Could you check a few things on this model? Use its own coordinates, in mm. A direction names the side the tool comes from. Round coordinates to 2 decimals unless told otherwise and drop trailing zeros. Write each loop counter-clockwise with the first axis right and the second up, starting at its lowest first coordinate (ties: lowest second). Pieces come first, ordered by that corner, then holes. Notation, with made-up numbers: (-4.5, 1.25) -> (30.5, 1.25) arc R30 ccw to (30.5, 25.25) -> close; hole circle Ø1 at (80.25, 61.5). An arc over 180 degrees is marked (long way). Answer as CSV lines item,"result". Start each with the question number.
Q1. For faces 4 (the flat face through (79, -133, 177)), 5 (the flat face through (-6.21, -167.31, 172.06)), 6 (the flat face through (77, -151, 0)), which set-ups out of +Z, -Z, +X, -X, +Y, -Y let a thin tool reach every point of the face, with its end or its side?
Q2. Imagine slicing it at C-C on y = -97. Please give me the cut outline in (x, z), and give its area (3 significant figures).
Q3. Imagine slicing it at B-B on z = 26.5. Please give me the cut outline in (x, y).
Q4. Imagine slicing it at A-A on x = 94. Please give me the cut outline in (y, z).
Q5. Will these pins go through, and if not, where does the flat tip stop? pin 1 Ø1 at (x, z) = (186.5, 194) entering from -Y; pin 2 Ø3 at (y, z) = (-92, 281.5) entering from -X; pin 3 Ø2 at (x, z) = (-22.5, 182.5) entering from -Y.
Q6. If we mould it in two halves opening along X, with no side actions, what happens to faces 1 (the flat face through (-47.62, -12.76, 172.06)), 2 (the flat face through (79, 0, 172)), 3 (the flat face through (186.5, -77, 177))? For each: pulls with the +X half, pulls with the -X half, needs draft (parallel to the pull), parting line crosses it, or undercut.
Q7. If I drill on line 1 (X direction, y = -88.5, z = 80); line 2 (X direction, y = -116, z = 50); line 3 (Y direction, x = 145, z = 61), over which ranges is the centre line in solid material (lowest first)? Write a range as [from, to].
Q8. Imagine slicing it at D-D on x = 232.5. Please give me the cut outline in (y, z).
Autodesk Inventor part; units mm, degrees
ref_plane "YZ Plane" through (0, 0, 0) normal (1, 0, 0) x (0, 1, 0)
ref_plane "XZ Plane" through (0, 0, 0) normal (0, 1, 0) x (-1, 0, 0)
ref_plane "XY Plane" through (0, 0, 0) normal (0, 0, 1) x (1, 0, 0)
sketch "Sketch1" plane through (0, 0, 0) normal (0, 0, 1) x (1, 0, 0)
  line L0 (0, 0) -> (160, 0)
  line L1 (160, 0) -> (118.589, -154.5481) construction
  line L2 (0, 0) -> (41.411, -154.5481) construction
  line L3 (41.411, -154.5481) -> (118.589, -154.5481)
  circle A0 centre (235.8871, -103.156) radius 80 construction
  line L4 (160, 0) -> (256.5926, -25.8819)
  line L5 (118.589, -154.5481) -> (215.1815, -180.43)
  arc A1 (215.1815, -180.43) -> (256.5926, -25.8819) centre (235.8871, -103.156) ccw
  circle A2 centre (-75.8871, -103.156) radius 80 construction
  line L6 (0, 0) -> (-96.5926, -25.8819)
  line L7 (41.411, -154.5481) -> (-55.1815, -180.43)
  arc A3 (-96.5926, -25.8819) -> (-55.1815, -180.43) centre (-75.8871, -103.156) ccw
  dimension "d0" = 160
  dimension "d1" = 160
  dimension "d2" = 160
  dimension "d3" = 75
  dimension "d4" = 75
  dimension "d5" = 160
  dimension "d6" = 100
  dimension "d7" = 160
  dimension "d9" = 100
extrude "Extrusion1" add sketch "Sketch1" along normal blind 349
sketch "Sketch2" plane through (0, 0, 349) normal (0, 0, 1) x (1, 0, 0)
  line L0 (-26.5, -133) -> (186.5, -133)
  line L1 (186.5, -133) -> (186.5, -20)
  line L2 (186.5, -20) -> (-26.5, -20)
  line L3 (-26.5, -20) -> (-26.5, -133)
  line L4 (160, 0) -> (0, 0)
  point P0 (80, -20)
  point P1 (80, 0)
  dimension "d12" = 213
  dimension "d13" = 113
  dimension "d14" = 20
extrude "Extrusion2" cut sketch "Sketch2" against normal through all
properties part number "Riser Base" material "ABS Plastic"
Checks:
1,face 4,"+Z, -Z"
1,face 5,"+Z, -Z, -Y"
1,face 6,"-Z, +X, -X, +Y, -Y"
2,outline,"(-155.65, 0) -> (-26.5, 0) -> (-26.5, 349) -> (-155.65, 349) -> close; (186.5, 0) -> (315.65, 0) -> (315.65, 349) -> (186.5, 349) -> close"
2,area,"90,100 mm^2"
3,outline,"(-96.59, -25.88) arc R80 ccw to (-55.18, -180.43) -> (41.41, -154.55) -> (118.59, -154.55) -> (215.18, -180.43) arc R80 ccw to (256.59, -25.88) -> (160, 0) -> (0, 0) -> close; hole (-26.5, -133) -> (186.5, -133) -> (186.5, -20) -> (-26.5, -20) -> close"
4,outline,"(-154.55, 0) -> (-133, 0) -> (-133, 349) -> (-154.55, 349) -> close; (-20, 0) -> (0, 0) -> (0, 349) -> (-20, 349) -> close"
5,pin 1,"y = -172.88"
5,pin 2,"x = -155.3"
5,pin 3,"y = -171.94"
6,face 1,"pulls with the -X half"
6,face 2,"needs draft"
6,face 3,"undercut"
7,line 1,"[-154.53, -26.5], [186.5, 314.53]"
7,line 2,"[-154.85, -26.5], [186.5, 314.85]"
7,line 3,"[-161.62, -133], [-20, 0]"
8,outline,"(-183.08, 0) -> (-19.43, 0) -> (-19.43, 349) -> (-183.08, 349) -> close"
